Here's how the part is built. I have some questions about the finished solid (model axes, mm). A direction names the side the tool comes from. Coordinates: 2 decimals unless noted, no trailing zeros. Order: outer loops, then holes, each group sorted by start corner. A loop starts at its lowest first (then second) coordinate and runs counter-clockwise, first axis right, second up. Notation, with made-up numbers: M 33.5,-36.75 L 82.5,-36.75 A17 cw 82.5,-23.75 Z; hole C 65,-19.5 d7. An arc over 180 degrees is marked long. One line per question, with ' | ' between items. Start each with the question number.
```python
from build123d import *

# Parameters (mm, degrees)
F0_R     = 11.3
F0_R_2   = 8.5
F1_DEPTH = 3
F0_W     = 40
F0_H     = 40
F2_DEPTH = 14
F3_R     = 4.7
F4_DEPTH = 40.001
F5_R     = 4.7
F5_R_2   = 2.4
F6_DEPTH = 5
F7_R     = 4.7
F7_R_2   = 2.4
F8_DEPTH = 5
F9_R     = 8
F10_R    = 1


with BuildPart() as f1:
    # F0 (on Top) → F1 (new body)
    with BuildSketch(Plane.XY):
        Circle(F0_R)
        Circle(F0_R_2, mode=Mode.SUBTRACT)
    extrude(amount=F1_DEPTH)

    # F0 (on Top) → F2 (join)
    with BuildSketch(Plane.XY):
        Rectangle(F0_W, F0_H)
        Circle(F0_R, mode=Mode.SUBTRACT)
    extrude(amount=F2_DEPTH)

    # F3 (on face) → F4 (cut, through all)
    with BuildSketch(Plane.XZ.offset(20)):
        with Locations((0, 8)):
            Circle(F3_R)
    extrude(amount=-F4_DEPTH, mode=Mode.SUBTRACT)

    # F5 (on face) → F6 (join)
    with BuildSketch(Plane.XZ.offset(20)):
        with Locations((0, 8)):
            Circle(F5_R)
        with Locations((0, 8)):
            Circle(F5_R_2, mode=Mode.SUBTRACT)
    extrude(amount=-F6_DEPTH)

    # F7 (on face) → F8 (join)
    with BuildSketch(Plane(origin=(0, 20, 0), x_dir=(-1, 0, 0), z_dir=(0, 1, 0))):
        with Locations((0, 8)):
            Circle(F7_R)
        with Locations((0, 8)):
            Circle(F7_R_2, mode=Mode.SUBTRACT)
    extrude(amount=-F8_DEPTH)

    # F9
    f9_edges = [f1.edges().sort_by_distance(p)[0] for p in [
        (-20, -20, 7),
        (-20, 20, 7),
        (20, -20, 7),
        (20, 20, 7),
    ]]
    fillet(f9_edges, radius=F9_R)

    # F10
    f10_edges = [f1.edges().sort_by_distance(p)[0] for p in [
        (0, -20, 14),
        (-11.3, 0, 14),
    ]]
    fillet(f10_edges, radius=F10_R)


solid = f1.part
```
1. Imagine slicing it at A-A (y = 0). List the corners of the cut face in (x, z) for me.
2. Imagine slicing it at D-D (z = 12). List the corners of the cut face in (x, y) for me, then the cut area to 3 significant figures.
3. I need wall thicknesses on line 1 (Z direction, x = 0, y = -18); line 2 (Y direction, x = 0, z = 11.5); line 3 (X direction, y = -10.5, z = 9.25). Which ranges of each line are inside material? Lowest first, please.
4. Imagine slicing it at B-B (z = 8). List the corners of the cut face in (x, y) for me.
5. Will these pins go through, and if not, where does the flat tip stop? pin 1 (8 mm diameter, centred on x = 16, y = 8, fed in from -Z); pin 2 (6 mm diameter, centred on x = -16, z = 6, fed in from +Y); pin 3 (4 mm diameter, centred on x = 15, z = 4, fed in from -Y); pin 4 (4.5 mm diameter, centred on x = 0, z = 8, fed in from +Y).
6. Which directions (+Z, -Z, +X, -X, +Y, -Y) give clear straight access to the entire face, cutting with the end or side of a thin tool? Please do faces 4 (the face through (-2, 15, 6)), 5 (the face through (10.438, -4.328, 7.93)), 6 (the face through (4.57, 7.167, 1.479)).
7. Imagine slicing it at C-C (x = 0). Count the separate pieces of the cut face and the enclosed holes in it, then the cut area to 3 significant figures.
8. We'd pull the mould along Y, two halves only. Please class faces 1 (the face through (2.53, 12.6, 11.96)), 2 (the face through (20, 0, 6)), 3 (the face through (17.594, -17.719, 6.591)): released by +Y, released by -Y, zero draft, split by the parting line, or undercut.
Entries:
1) outline: M -20,0 L -8.5,0 L -8.5,3 L -11.3,3 L -11.3,13 A1 ccw -12.3,14 L -19,14 A1 ccw -20,13 Z; M 8.5,0 L 20,0 L 20,13 A1 ccw 19,14 L 12.3,14 A1 ccw 11.3,13 L 11.3,3 L 8.5,3 Z
2) outline: M -20,-12 A8 ccw -12,-20 L 12,-20 A8 ccw 20,-12 L 20,12 A8 ccw 12,20 L -12,20 A8 ccw -20,12 Z; hole M -2.47,-15 L 2.47,-15 L 2.47,-11.03 A11.3 ccw 2.47,11.03 L 2.47,15 L -2.47,15 L -2.47,11.03 A11.3 ccw -2.47,-11.03 Z | area: 1,110 mm²
3) line 1: 0 to 5.6, 10.4 to 14 | line 2: -20 to -15, 15 to 20 | line 3: -20 to -4.53, 4.53 to 20
4) outline: M -20,-12 A8 ccw -12,-20 L -2.4,-20 L -2.4,-15 L -4.7,-15 L -4.7,-10.28 A11.3 cw -4.7,10.28 L -4.7,15 L -2.4,15 L -2.4,20 L -12,20 A8 ccw -20,12 Z; M 2.4,-20 L 12,-20 A8 ccw 20,-12 L 20,12 A8 ccw 12,20 L 2.4,20 L 2.4,15 L 4.7,15 L 4.7,10.28 A11.3 cw 4.7,-10.28 L 4.7,-15 L 2.4,-15 Z
5) pin 1: z = 0 | pin 2: y = 19.94 | pin 3: y = -19.94 | pin 4: through
6) face 4: none | face 5: +Z | face 6: +Z, -Z
7) separate pieces: 4 | enclosed holes: 0 | area: 142 mm²
8) face 1: undercut | face 2: zero draft | face 3: released by -Y
